```python
from build123d import *

# Parameters (mm, degrees)
SKETCH_1_R      = 2.55
EXTRUDE_1_DEPTH = 180
FILLET_1_R      = 1


with BuildPart() as part:
    # 草图1 → 凸台-拉伸1 (new body)
    with BuildSketch(Plane.XY):
        Polygon((4.62194142, 1.905266374), (6.694733626, 3.97805858), (6.694733626, 6.205266374), (5.094733626, 6.205266374), (5.094733626, 8.005266374), (11.994733626, 8.005266374), (11.994733626, 1.105266374), (10.194733626, 1.105266374), (10.194733626, 2.705266374), (7.967525833, 2.705266374), (5.894733626, 0.632474167), (5.894733626, -4.62194142), (7.967525833, -6.694733626), (10.194733626, -6.694733626), (10.194733626, -5.094733626), (11.994733626, -5.094733626), (11.994733626, -11.994733626), (5.094733626, -11.994733626), (5.094733626, -10.194733626), (6.694733626, -10.194733626), (6.694733626, -7.967525833), (4.62194142, -5.894733626), (-0.632474167, -5.894733626), (-2.705266374, -7.967525833), (-2.705266374, -10.194733626), (-1.105266374, -10.194733626), (-1.105266374, -11.994733626), (-8.005266374, -11.994733626), (-8.005266374, -5.094733626), (-6.205266374, -5.094733626), (-6.205266374, -6.694733626), (-3.97805858, -6.694733626), (-1.905266374, -4.62194142), (-1.905266374, 0.632474167), (-3.97805858, 2.705266374), (-6.205266374, 2.705266374), (-6.205266374, 1.105266374), (-8.005266374, 1.105266374), (-8.005266374, 8.005266374), (-1.105266374, 8.005266374), (-1.105266374, 6.205266374), (-2.705266374, 6.205266374), (-2.705266374, 3.97805858), (-0.632474167, 1.905266374), align=None)
        with Locations(Location((1.994733626, -1.994733626, 0), (0, 0, 180))):
            Circle(SKETCH_1_R, mode=Mode.SUBTRACT)
    extrude(amount=EXTRUDE_1_DEPTH)

    # 圆角1
    fillet_1_edges = [part.edges().sort_by_distance(p)[0] for p in [
        (-8.005266374, -11.994733626, 90),
        (-8.005266374, 8.005266374, 90),
        (11.994733626, 8.005266374, 90),
        (11.994733626, -11.994733626, 90),
    ]]
    fillet(fillet_1_edges, radius=FILLET_1_R)


solid = part.part
```
The model under review builds one solid part; all positions refer to its coordinate system, in mm. A direction names the side the tool comes from. Give positions to 0.01 mm unless a question says otherwise; leave off trailing zeros. Write each loop counter-clockwise with the first axis right and the second up, starting at its lowest first coordinate (ties: lowest second). Pieces come first, ordered by that corner, then holes. Notation, with made-up numbers: M 89.25,-3.75 L 128.25,-3.75 A6 cw 128.25,4.25 Z; hole C 60,5 d9. An arc over 180 degrees is marked long. Write each question's results on one line, items separated by ' | '. Start each with the question number.
1. Insertion check: pin 1 Ø2 at (x, y) = (3.5, 3) entering from +Z; pin 2 Ø1 at (x, y) = (-4.5, -9.5) entering from -Z; pin 3 Ø4 at (y, z) = (-2.5, 124.5) entering from -X. Each pin has a flat end and moves straight along its axis. Give the tip position at first contact, or say it passes through.
2. For probe 1 along Y at (x, z) = (-5.5, 33); probe 2 along X at (y, z) = (6, 171); probe 3 along X at (y, z) = (-10.5, 147), list the stretches that pass through material, from the lowest coordinate up. Write a range as [from, to].
3. For faces 5 (the flat face through (11.995, 4, 89)), 6 (the flat face through (5.895, -2, 89)), list the 3-axis set-ups (+Z, -Z, +X, -X, +Y, -Y) from which the entire face can be reached by the end or side of a thin tool; tool diameter is ignored.
4. We need section A-A (x = 2). Write out the cut boundary in (y, z), and give its area (3 significant figures).
5. Mouldability with a two-part tool opening along Y and no side actions: class faces 1 (the flat face through (2, -5.895, 89)), 2 (the flat face through (4, 0, 180)), 3 (the flat face through (2, 1.905, 89)), 4 (the flat face through (-1.905, -2, 89)) as released by +Y, released by -Y, zero draft, split by the parting line, or undercut.
Results found:
1) pin 1: passes through | pin 2: stops at z = 0 | pin 3: stops at x = -1.91
2) probe 1: y = [-11.99, -6.69], [2.71, 8.01] | probe 2: x = [-8.01, -2.71], [6.69, 11.99] | probe 3: x = [-8.01, -1.11], [5.09, 11.99]
3) face 5: +Z, -Z, +X, +Y, -Y | face 6: +Z, -Z, +X
4) outline: M -5.89,0 L -4.54,0 L -4.54,180 L -5.89,180 Z; M 0.56,0 L 1.91,0 L 1.91,180 L 0.56,180 Z | area: 486 mm^2
5) face 1: released by -Y | face 2: zero draft | face 3: released by +Y | face 4: undercut
